Read the model definition and answer for the solid it produces. Units are mm, in the model's axes. Face numbers are marked on the shaded views. A direction names the side the tool comes from. Coordinates: 2 decimals unless noted, no trailing zeros. Loops run counter-clockwise (first coordinate to the right, second up) from the corner with the lowest first, then second, coordinate; pieces in that order, holes last. Notation, with made-up numbers: (27, 17) - (58, 17) arc R20 ccw to (58, 36) - close; hole circle Ø3 at (6.25, 4). An arc over 180 degrees is marked (long way). Use CSV: the item, a comma, the result in double quotes.
```python
from build123d import *

# Parameters (mm, degrees)
BOSS_EXTRUDE1_DEPTH = 35
SHELL1_T            = 2
SKETCH2_R           = 4
BOSS_EXTRUDE2_DEPTH = 35
FILLET2_START       = -1
FILLET2_DEPTH       = 36


with BuildPart() as part:
    # Sketch1 → Boss-Extrude1 (new body)
    with BuildSketch(Plane.XY):
        with BuildLine():
            Line((-51, -31), (51, -31))
            ThreePointArc((51, -31), (53.828427125, -29.828427125), (55, -27))
            Line((55, -27), (55, 27))
            ThreePointArc((55, 27), (53.828427125, 29.828427125), (51, 31))
            Line((51, 31), (-51, 31))
            ThreePointArc((-51, 31), (-53.828427125, 29.828427125), (-55, 27))
            Line((-55, 27), (-55, -27))
            ThreePointArc((-55, -27), (-53.828427125, -29.828427125), (-51, -31))
        make_face()
    extrude(amount=BOSS_EXTRUDE1_DEPTH)

    # Shell1
    shell1_openings = [part.faces().sort_by_distance(p)[0] for p in [
        (0, 0, 35),
    ]]
    offset(amount=SHELL1_T, openings=shell1_openings, kind=Kind.INTERSECTION)

    # Sketch2 → Boss-Extrude2 (add)
    with BuildSketch(Plane.XY):
        with Locations((-51, 27)):
            Circle(SKETCH2_R)
        with Locations((51, 27)):
            Circle(SKETCH2_R)
        with Locations((51, -27)):
            Circle(SKETCH2_R)
        with Locations((-51, -27)):
            Circle(SKETCH2_R)
    extrude(amount=BOSS_EXTRUDE2_DEPTH)

    # Fillet2: read off the stored shape, not the designer's step
    # Fillet2 outline → Fillet2 (add)
    with BuildSketch(Plane.XY.offset(FILLET2_START)):
        with BuildLine():
            ThreePointArc((51, -31), (48.381385317, -30.023715784), (47.041026725, -27.571428571))
            ThreePointArc((47.041026725, -27.571428571), (46.339583608, -29.963961012), (44.07179677, -31))
            Line((44.07179677, -31), (51, -31))
        make_face()
        with BuildLine():
            ThreePointArc((55, -20.07179677), (53.963961012, -22.339583608), (51.571428571, -23.041026726))
            ThreePointArc((51.571428571, -23.041026726), (54.023715784, -24.381385317), (55, -27))
            Line((55, -27), (55, -20.07179677))
        make_face()
        with BuildLine():
            Line((-51, -31), (-44.07179677, -31))
            ThreePointArc((-44.07179677, -31), (-46.339583608, -29.963961012), (-47.041026726, -27.571428571))
            ThreePointArc((-47.041026726, -27.571428571), (-48.381385317, -30.023715784), (-51, -31))
        make_face()
        with BuildLine():
            ThreePointArc((51.571428571, 23.041026726), (53.963961012, 22.339583608), (55, 20.07179677))
            Line((55, 20.07179677), (55, 27))
            ThreePointArc((55, 27), (54.023715784, 24.381385317), (51.571428571, 23.041026726))
        make_face()
        with BuildLine():
            ThreePointArc((-55, -27), (-54.023715784, -24.381385317), (-51.571428571, -23.041026725))
            ThreePointArc((-51.571428571, -23.041026725), (-53.963961012, -22.339583608), (-55, -20.07179677))
            Line((-55, -20.07179677), (-55, -27))
        make_face()
        with BuildLine():
            ThreePointArc((44.07179677, 31), (46.339583608, 29.963961012), (47.041026726, 27.571428571))
            ThreePointArc((47.041026726, 27.571428571), (48.381385317, 30.023715784), (51, 31))
            Line((51, 31), (44.07179677, 31))
        make_face()
        with BuildLine():
            Line((-55, 27), (-55, 20.07179677))
            ThreePointArc((-55, 20.07179677), (-53.963961012, 22.339583608), (-51.571428571, 23.041026726))
            ThreePointArc((-51.571428571, 23.041026726), (-54.023715784, 24.381385317), (-55, 27))
        make_face()
        with BuildLine():
            ThreePointArc((-47.041026726, 27.571428571), (-46.339583608, 29.963961012), (-44.07179677, 31))
            Line((-44.07179677, 31), (-51, 31))
            ThreePointArc((-51, 31), (-48.381385317, 30.023715784), (-47.041026726, 27.571428571))
        make_face()
    extrude(amount=FILLET2_DEPTH)


solid = part.part
```
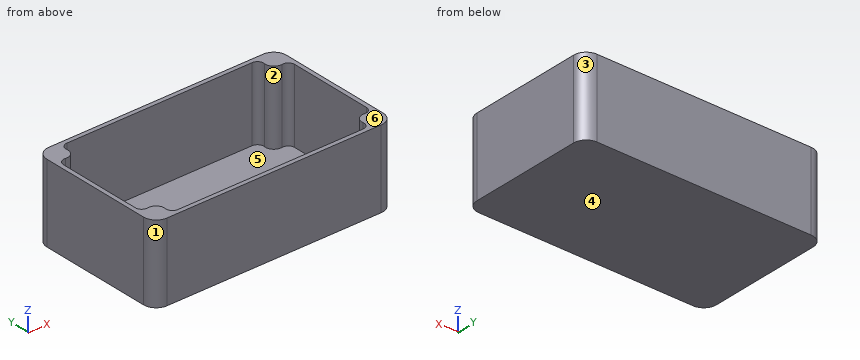
Q1. Given P1, Ø5, axis at x = -22.5, y = 25, coming from the +Z side, flat-ended and moving along its own axis, determine where the tip first touches the part or whether it passes through.
Reported:
P1,"stops at z = 0"
Q2. The part is cut by section A-A on x = 36.5. Determine the outline of the cut face in (y, z).
Reported:
outline,"(-33, -2) - (33, -2) - (33, 35) - (31, 35) - (31, 0) - (-31, 0) - (-31, 35) - (-33, 35) - close"
Q3. The part is cut by section C-C on y = -8. Determine the outline of the cut face in (x, z), and give its area (3 significant figures).
Reported:
outline,"(-57, -2) - (57, -2) - (57, 35) - (55, 35) - (55, 0) - (-55, 0) - (-55, 35) - (-57, 35) - close"
area,"368 mm²"
Q4. For a pull along X with two mould halves and no side action, classify the marked faces 1, 2, 3 and 4 as +X half, -X half, draft (parallel to the pull), parting line (faces both ways), or undercut.
Reported:
face 1,"-X half"
face 2,"undercut"
face 3,"+X half"
face 4,"draft"
Q5. The part is cut by section B-B on z = 33.5. Determine the outline of the cut face in (x, y).
Reported:
outline,"(-57, -27) arc R6 ccw to (-51, -33) - (51, -33) arc R6 ccw to (57, -27) - (57, 27) arc R6 ccw to (51, 33) - (-51, 33) arc R6 ccw to (-57, 27) - close; hole (-55, -20.07) arc R3 ccw to (-51.57, -23.04) arc R4 cw to (-47.04, -27.57) arc R3 ccw to (-44.07, -31) - (44.07, -31) arc R3 ccw to (47.04, -27.57) arc R4 cw to (51.57, -23.04) arc R3 ccw to (55, -20.07) - (55, 20.07) arc R3 ccw to (51.57, 23.04) arc R4 cw to (47.04, 27.57) arc R3 ccw to (44.07, 31) - (-44.07, 31) arc R3 ccw to (-47.04, 27.57) arc R4 cw to (-51.57, 23.04) arc R3 ccw to (-55, 20.07) - close"
Q6. Find the intervals of material crossed by probe 1 along Y at (x, z) = (30, 16); probe 2 along X at (y, z) = (-9.5, 28.5); probe 3 along Z at (x, y) = (8, 2), in increasing order. Write a range as [from, to].
Reported:
probe 1,"y = [-33, -31], [31, 33]"
probe 2,"x = [-57, -55], [55, 57]"
probe 3,"z = [-2, 0]"
Q7. A tool of negligible diameter and unlimited length cuts with its end or side. For the marked faces 5 and 6, from which of +Z, -Z, +X, -X, +Y, -Y can it reach the whole face along a straight path? Write none if from no direction.
Reported:
face 5,"+Z"
face 6,"+Z, +X, -X, +Y, -Y"
